Can you work these out from the model? Positions are in its coordinate system, mm. A direction names the side the tool comes from. Round coordinates to 2 decimals unless told otherwise and drop trailing zeros. Loops run counter-clockwise (first coordinate to the right, second up) from the corner with the lowest first, then second, coordinate; pieces in that order, holes last. Notation, with made-up numbers: M 84,15.5 L 111,15.5 A24 cw 111,29.5 Z; hole C 2,78.25 d6. An arc over 180 degrees is marked long. Use a Markdown table: item, result. Add a question column.
```python
from build123d import *


with BuildPart() as part:
    # Revolve profile 1 → Revolve 1 (revolve)
    with BuildSketch(Plane(origin=(0, 0, 0), x_dir=(1, 0, 0), z_dir=(0, 1, 0)), mode=Mode.PRIVATE) as revolve_1_sk:
        Polygon((0, -300), (0, 0), (12.5, 0), (14, -2), (14, -16), (16, -19), (16, -232), (17, -234), (17, -270), (11, -273), (11, -300), align=None)
    revolve(revolve_1_sk.sketch.rotate(Axis((0, 0, -5), (0, 0, 1)), 180), axis=Axis((0, 0, -5), (0, 0, 1)))


solid = part.part
```
(1) Suppose I cut it at A-A on y = 0. List the corners of the cut face in (x, z) for me, and give its area (3 significant figures).
(2) Suppose I cut it at C-C on z = 124. List the corners of the cut face in (x, y) for me, and give its area (3 significant figures).
(3) I'm going to push flat-ended pins straight in: pin 1 (5 mm diameter, centred on y = -6, z = 34, fed in from -X); pin 2 (3 mm diameter, centred on x = -13.5, y = 4.5, fed in from +Z); pin 3 (6 mm diameter, centred on x = 2.5, z = 192.5, fed in from +Y). Where does each tip first touch, or does it pass through?
(4) On a 3-axis mill with a long thin cutter (end or side, diameter ignored), from which of +Z, -Z, +X, -X, +Y, -Y can I reach the whole of each face in a straight line? I mean faces 1 (the face through (3.47, 15.62, 126.99)), 2 (the face through (0, 0, 300)), 3 (the face through (2.38, 10.74, 286.69)). Say none if no direction works.
(5) If I drill on probe 1 along X at (y, z) = (-0.5, 251); probe 2 along Y at (x, z) = (7, 269.5); probe 3 along Y at (x, z) = (0.5, 65), over which ranges is the centre line in solid material (lowest first)? Write a range as [from, to].
Results below:
| question | item | result |
|---|---|---|
| 1 | outline | M -17,234 L -16,232 L -16,19 L -14,16 L -14,2 L -12.5,0 L 12.5,0 L 14,2 L 14,16 L 16,19 L 16,232 L 17,234 L 17,270 L 11,273 L 11,300 L -11,300 L -11,273 L -17,270 Z |
| 1 | area | 9,320 mm² |
| 2 | outline | C 0,0 d32 |
| 2 | area | 804 mm² |
| 3 | pin 1 | stops at x = -15.61 |
| 3 | pin 2 | stops at z = 272.13 |
| 3 | pin 3 | stops at y = 16 |
| 4 | face 1 | -Z |
| 4 | face 2 | +Z, +X, -X, +Y, -Y |
| 4 | face 3 | +Z |
| 5 | probe 1 | x = [-16.99, 16.99] |
| 5 | probe 2 | y = [-15.49, 15.49] |
| 5 | probe 3 | y = [-15.99, 15.99] |
